Here's how the part is built. I have some questions about the finished solid (model axes, mm). A direction names the side the tool comes from. Round coordinates to 2 decimals unless told otherwise and drop trailing zeros. Order: outer loops, then holes, each group sorted by start corner. A loop starts at its lowest first (then second) coordinate and runs counter-clockwise, first axis right, second up. Notation, with made-up numbers: M 16.5,35.5 L 45.5,35.5 A8 cw 45.5,45.5 Z; hole C -10.5,60.5 d11. An arc over 180 degrees is marked long. Use one line per item in the form item = value. Start each with the question number.
```python
from build123d import *

# Parameters (mm, degrees)
FILLET2_R = 0.254


with BuildPart() as part:
    # Sketch1 → Revolve1 (revolve)
    with BuildSketch(Plane(origin=(0, 0, 0), x_dir=(0, 0, -1), z_dir=(1, 0, 0)), mode=Mode.PRIVATE) as revolve1_sk:
        Polygon((7.541506618, 1.11125), (20.9296, 1.11125), (20.9296, 1.6764), (17.826604011, 2.0574), (17.506907051, 1.6764), (14.403911062, 2.0574), (14.084214103, 1.6764), (8.2296, 1.6764), (8.2296, 3.7338), (3.4544, 3.7338), (3.4544, 4.6609), (3.3274, 4.7879), (0, 4.7879), (0, 3.9751), (1.061768562, 3.175), (6.35, 3.175), align=None)
    revolve(revolve1_sk.sketch.rotate(Axis((0, 0, -9.412698919), (0, 0, -1)), 90), axis=Axis((0, 0, -9.412698919), (0, 0, -1)))

    # Fillet2
    fillet2_edges = [part.edges().sort_by_distance(p)[0] for p in [
        (-3.7338, 0, -8.2296),
        (-1.6764, 0, -20.9296),
    ]]
    fillet(fillet2_edges, radius=FILLET2_R)


solid = part.part
```
1) If we section it at A-A on z = -11.25: Write out the boundary of the cut face in (x, y).
2) If we mould it in two halves opening along Z, with no side actions, what happens to faces 5 (the flat face through (0, -4, -3.454)), 6 (the conical face through (0.843, 1.621, -16.278)), 7 (the cylindrical face through (0.77, 1.49, -11.12)), 8 (the flat face through (-2, -4, 0))? For each: +Z half, -Z half, draft (parallel to the pull), parting line (faces both ways), or undercut.
3) On a 3-axis mill with a long thin cutter (end or side, diameter ignored), from which of +Z, -Z, +X, -X, +Y, -Y can I reach the whole of each face in a straight line? I mean faces 1 (the flat face through (2, 1, -8.23)), 2 (the cylindrical face through (-2.52, 1.93, -3.74)), 3 (the cylindrical face through (-0.241, 1.085, -14.329)), 4 (the cylindrical face through (-0.809, 3.645, -5.683)). Say none if no direction works.
4) If I drill on line 1 (Y direction, x = 0, z = -2.5) (3 decimals); line 2 (Y direction, x = 0, z = -3.7) (3 decimals); line 3 (X direction, y = 0.25, z = -1.5), over which ranges is the centre line in solid material (lowest first)?
5) Will these pins go through, and if not, where does the flat tip stop? pin 1 Ø4 at (y, z) = (-2.5, -15) entering from -X; pin 2 Ø1.5 at (x, y) = (-3.5, 1) entering from -Z; pin 3 Ø2 at (y, z) = (-2, -9.5) entering from +X.
Completed:
q1.outline = C 0,0 d3.35; hole C 0,0 d2.22
q2.face_5 = -Z half
q2.face_6 = undercut
q2.face_7 = undercut
q2.face_8 = +Z half
q3.face_1 = none
q3.face_2 = +Z
q3.face_3 = +Z, -Z
q3.face_4 = -Z
q4.line_1 = -4.788 to -3.175, 3.175 to 4.788
q4.line_2 = -3.734 to -3.175, 3.175 to 3.734
q4.line_3 = -4.78 to -3.17, 3.17 to 4.78
q5.pin_1 = -1.97
q5.pin_2 = -8.23
q5.pin_3 = 1.35
